Check sheet for the modelled part. Datum: model origin and axes. Units: mm. Face numbers are marked on the shaded views. Give positions to 0.01 mm unless a question says otherwise; leave off trailing zeros. Order: outer loops, then holes, each group sorted by start corner. A loop starts at its lowest first (then second) coordinate and runs counter-clockwise, first axis right, second up. Notation, with made-up numbers: M 18,50.5 L 37,50.5 A25 ccw 37,86.5 Z; hole C -13,-14.5 d4. An arc over 180 degrees is marked long. Answer in a Markdown table with one row per item. Add a question column.
from build123d import *

# Parameters (mm, degrees)
SKETCH1_W                                  = 250
SKETCH1_H                                  = 250
BOSS_EXTRUDE1_DEPTH                        = 25
SKETCH2_W                                  = 230
SKETCH2_H                                  = 230
CUT_EXTRUDE1_DEPTH                         = 25
SKETCH19_W                                 = 41
SKETCH19_H                                 = 21
CUT_EXTRUDE10_DEPTH                        = 9.3
SKETCH20_R                                 = 5
CUT_EXTRUDE11_DEPTH                        = 9.3
SKETCH23_W                                 = 49
SKETCH23_H                                 = 1.1
CUT_EXTRUDE14_DEPTH                        = 1
SKETCH21_R                                 = 1.125
CUT_EXTRUDE12_DEPTH                        = 10
MIRROR1_AT_THE_SECOND_PLANE_COPY_1_SKETC_R = 1.125
MIRROR1_AT_THE_SECOND_PLANE_COPY_1_DEPTH   = 10
MIRROR2_COPY_1_SKETCH_R                    = 1.125
MIRROR2_COPY_1_DEPTH                       = 10
MIRROR2_COPY_2_SKETCH_R                    = 1.125
MIRROR2_COPY_2_DEPTH                       = 10
MIRROR2_COPY_3_SKETCH_R                    = 1.125
MIRROR2_COPY_3_DEPTH                       = 10
SKETCH22_R                                 = 2.5
CUT_EXTRUDE13_DEPTH                        = 281.624304008


with BuildPart() as part:
    # Sketch1 → Boss-Extrude1 (new body)
    with BuildSketch(Plane(origin=(0, 0, 0), x_dir=(1, 0, 0), z_dir=(0, 1, 0))):
        Rectangle(SKETCH1_W, SKETCH1_H)
    extrude(amount=BOSS_EXTRUDE1_DEPTH)

    # Sketch2 → Cut-Extrude1 (cut)
    with BuildSketch(Plane(origin=(0, 25, 0), x_dir=(1, 0, 0), z_dir=(0, 1, 0))):
        Rectangle(SKETCH2_W, SKETCH2_H)
    extrude(amount=-CUT_EXTRUDE1_DEPTH, mode=Mode.SUBTRACT)

    # Sketch19 → Cut-Extrude10 (cut)
    with BuildSketch(Plane.ZY.offset(125)):
        with Locations((10.5, 12.5)):
            Rectangle(SKETCH19_W, SKETCH19_H)
    cut_extrude10 = extrude(amount=-CUT_EXTRUDE10_DEPTH, mode=Mode.SUBTRACT)

    # Sketch20 → Cut-Extrude11 (cut)
    with BuildSketch(Plane.ZY.offset(115.7)):
        with Locations((0, 12.5)):
            Circle(SKETCH20_R)
    cut_extrude11 = extrude(amount=-CUT_EXTRUDE11_DEPTH, mode=Mode.SUBTRACT)

    # Sketch23 → Cut-Extrude14 (cut)
    with BuildSketch(Plane.ZY.offset(125)):
        with Locations((10.5, 12.5)):
            Rectangle(SKETCH23_W, SKETCH23_H)
    cut_extrude14 = extrude(amount=-CUT_EXTRUDE14_DEPTH, mode=Mode.SUBTRACT)

    # Sketch21 → Cut-Extrude12 (cut)
    with BuildSketch(Plane.ZY.offset(125)):
        with Locations((-13.9, 17.6)):
            Circle(SKETCH21_R)
    cut_extrude12 = extrude(amount=-CUT_EXTRUDE12_DEPTH, mode=Mode.SUBTRACT)

    # Mirror1: Cut-Extrude12 across plane
    add(cut_extrude12.mirror(Plane.XY.offset(10.5)), mode=Mode.SUBTRACT)

    # Mirror1 at the second plane: Cut-Extrude12 across plane
    add(cut_extrude12.mirror(Plane.ZX.offset(12.5)), mode=Mode.SUBTRACT)

    # Mirror1 at the second plane copy 1 sketc → Mirror1 at the second plane copy 1 (cut)
    with BuildSketch(Plane(origin=(-125, 25, 21), x_dir=(0, 0, -1), z_dir=(-1, 0, 0))):
        with Locations((-13.9, 17.6)):
            Circle(MIRROR1_AT_THE_SECOND_PLANE_COPY_1_SKETC_R)
    extrude(amount=-MIRROR1_AT_THE_SECOND_PLANE_COPY_1_DEPTH, mode=Mode.SUBTRACT)

    # Mirror2: Cut-Extrude10, Cut-Extrude11, Cut-Extrude14, Cut-Extrude12 across plane
    add(cut_extrude10.mirror(Plane.ZY), mode=Mode.SUBTRACT)
    add(cut_extrude11.mirror(Plane.ZY), mode=Mode.SUBTRACT)
    add(cut_extrude14.mirror(Plane.ZY), mode=Mode.SUBTRACT)
    add(cut_extrude12.mirror(Plane.ZY), mode=Mode.SUBTRACT)

    # Mirror2 copy 1 sketch → Mirror2 copy 1 (cut)
    with BuildSketch(Plane(origin=(125, 0, 21), x_dir=(0, 0, -1), z_dir=(1, 0, 0))):
        with Locations((-13.9, 17.6)):
            Circle(MIRROR2_COPY_1_SKETCH_R)
    extrude(amount=-MIRROR2_COPY_1_DEPTH, mode=Mode.SUBTRACT)

    # Mirror2 copy 2 sketch → Mirror2 copy 2 (cut)
    with BuildSketch(Plane(origin=(125, 25, 0), x_dir=(0, 0, 1), z_dir=(1, 0, 0))):
        with Locations((-13.9, 17.6)):
            Circle(MIRROR2_COPY_2_SKETCH_R)
    extrude(amount=-MIRROR2_COPY_2_DEPTH, mode=Mode.SUBTRACT)

    # Mirror2 copy 3 sketch → Mirror2 copy 3 (cut)
    with BuildSketch(Plane(origin=(125, 25, 21), x_dir=(0, 0, -1), z_dir=(1, 0, 0))):
        with Locations((-13.9, -17.6)):
            Circle(MIRROR2_COPY_3_SKETCH_R)
    extrude(amount=-MIRROR2_COPY_3_DEPTH, mode=Mode.SUBTRACT)

    # Sketch22 → Cut-Extrude13 (cut, through all)
    with BuildSketch(Plane.XY.offset(125)):
        with Locations((-20, 12.5)):
            Circle(SKETCH22_R)
        with Locations((20, 12.5)):
            Circle(SKETCH22_R)
    extrude(amount=-CUT_EXTRUDE13_DEPTH, mode=Mode.SUBTRACT)


solid = part.part
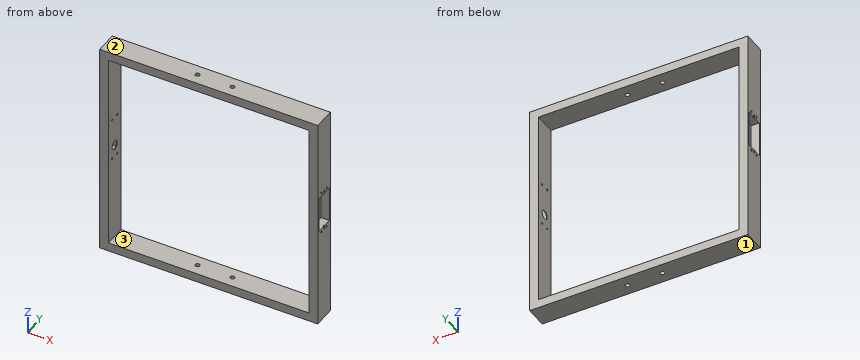
Q1. Cross-section at A-A (z = 63.5). Record the boundary of the cut face in (x, y), and give its area (3 significant figures).
Q2. Draft check along Z on the marked faces 1, 2 and 3. Enter one of: pulls with the +Z half, pulls with the -Z half, needs draft (parallel to the pull), parting line crosses it, or undercut.
Q3. Thickness scan on probe 1 along Y at (x, z) = (-121, -13.9) (3 decimals); probe 2 along Z at (x, y) = (-121.5, 7.4) (3 decimals); probe 3 along X at (y, z) = (15.75, -100.5). Record the ranges inside material, lowest first.
Q4. Cross-section at B-B (x = -6). Record the boundary of the cut face in (y, z), and give its area (3 significant figures).
Q5. Cross-section at C-C (z = 0). Record the boundary of the cut face in (x, y).
Q6. Go/stop test with flat-tipped pins: pin 1 (13 mm diameter, centred on y = 12.5, z = 0, fed in from -X); pin 2 (1.5 mm diameter, centred on y = 14.5, z = 3.5, fed in from -X) (3 decimals). Record where each tip stops, or that it passes through.
Values follow:
| question | item | result |
|---|---|---|
| 1 | outline | M -125,0 L -115,0 L -115,25 L -125,25 Z; M 115,0 L 125,0 L 125,25 L 115,25 Z |
| 1 | area | 500 mm² |
| 2 | face 1 | pulls with the -Z half |
| 2 | face 2 | pulls with the +Z half |
| 2 | face 3 | undercut |
| 3 | probe 1 | 0 to 6.275, 8.525 to 16.475, 18.725 to 25 |
| 3 | probe 2 | -125 to -15.025, -12.775 to -10, 31 to 33.775, 36.025 to 125 |
| 3 | probe 3 | -125 to -115, 115 to 125 |
| 4 | outline | M 0,-125 L 25,-125 L 25,-115 L 0,-115 Z; M 0,115 L 25,115 L 25,125 L 0,125 Z |
| 4 | area | 500 mm² |
| 5 | outline | M -125,0 L -115,0 L -115,7.5 L -115.7,7.5 L -115.7,2 L -125,2 Z; M -125,23 L -115.7,23 L -115.7,17.5 L -115,17.5 L -115,25 L -125,25 Z; M 115,0 L 125,0 L 125,2 L 115.7,2 L 115.7,7.5 L 115,7.5 Z; M 115,17.5 L 115.7,17.5 L 115.7,23 L 125,23 L 125,25 L 115,25 Z |
| 6 | pin 1 | x = -115.7 |
| 6 | pin 2 | through |
